from build123d import *

# Parameters (mm, degrees)
SKETCH1_W               = 20
SKETCH1_H               = 40
BOSS_EXTRUDE1_DEPTH     = 20
SKETCH2_W               = 13.1
SKETCH2_H               = 13.1
CUT_EXTRUDE1_DEPTH      = 49.989794856
SKETCH3_W               = 13.1
SKETCH3_H               = 13.1
CUT_EXTRUDE2_DEPTH      = 40.033447196
BOSS_EXTRUDE2_DEPTH     = 10
SKETCH5_W               = 20
SKETCH5_H               = 40
BOSS_EXTRUDE3_DEPTH     = 12
SKETCH6_W               = 13.1
SKETCH6_H               = 8
CUT_EXTRUDE3_DEPTH      = 13.1
SKETCH7_R               = 2
CUT_EXTRUDE4_DEPTH      = 55.990908339
CUT_EXTRUDE5_DEPTH      = 54.83216975
CUT_EXTRUDE5_DEPTH_BACK = 54.83216975
SKETCH8_R               = 2
CUT_EXTRUDE6_DEPTH      = 55.990908339


with BuildPart() as part:
    # Sketch1 → Boss-Extrude1 (new body)
    with BuildSketch(Plane(origin=(0, 0, 0), x_dir=(1, 0, 0), z_dir=(0, 1, 0))):
        with Locations((10, 20)):
            Rectangle(SKETCH1_W, SKETCH1_H)
    extrude(amount=BOSS_EXTRUDE1_DEPTH)

    # Sketch2 → Cut-Extrude1 (cut, through all)
    with BuildSketch(Plane(origin=(0, 20, 0), x_dir=(1, 0, 0), z_dir=(0, 1, 0))):
        with Locations((10, 6.55)):
            Rectangle(SKETCH2_W, SKETCH2_H)
    extrude(amount=-CUT_EXTRUDE1_DEPTH, mode=Mode.SUBTRACT)

    # Sketch3 → Cut-Extrude2 (cut, through all)
    with BuildSketch(Plane.XY.offset(-13.1)):
        with Locations((10, 13.45)):
            Rectangle(SKETCH3_W, SKETCH3_H)
    extrude(amount=-CUT_EXTRUDE2_DEPTH, mode=Mode.SUBTRACT)

    # Sketch4 → Boss-Extrude2 (add)
    with BuildSketch(Plane.XZ):
        Polygon((3.45, -13.1), (3.45, 0), (0, 0), (0, -40), (20, -40), (20, 0), (16.55, 0), (16.55, -13.1), align=None)
    extrude(amount=BOSS_EXTRUDE2_DEPTH)

    # Sketch5 → Boss-Extrude3 (add)
    with BuildSketch(Plane(origin=(0, 20, 0), x_dir=(1, 0, 0), z_dir=(0, 1, 0))):
        with Locations((10, 20)):
            Rectangle(SKETCH5_W, SKETCH5_H)
    extrude(amount=BOSS_EXTRUDE3_DEPTH)

    # Sketch6 → Cut-Extrude3 (cut)
    with BuildSketch(Plane.XY):
        with Locations((10, 24)):
            Rectangle(SKETCH6_W, SKETCH6_H)
    extrude(amount=-CUT_EXTRUDE3_DEPTH, mode=Mode.SUBTRACT)

    # Sketch7 → Cut-Extrude4 (cut, through all)
    with BuildSketch(Plane(origin=(20, 0, 0), x_dir=(0, 0, -1), z_dir=(1, 0, 0))):
        with Locations((6.55, -4)):
            Circle(SKETCH7_R)
        with Locations((6.55, 16)):
            Circle(SKETCH7_R)
        with Locations((6.55, 6)):
            Circle(SKETCH7_R)
    extrude(amount=-CUT_EXTRUDE4_DEPTH, mode=Mode.SUBTRACT)

    # Sketch8 → Cut-Extrude5 (cut, two sides: drawn at the far end of the back side and taken through both)
    with BuildSketch(Plane(origin=(3.45, 0, 0), x_dir=(0, 0, -1), z_dir=(1, 0, 0)).offset(-CUT_EXTRUDE5_DEPTH_BACK)):
        with Locations((34, 13.45)):
            Circle(SKETCH8_R)
        with Locations((26, 13.45)):
            Circle(SKETCH8_R)
        with Locations((18, 13.45)):
            Circle(SKETCH8_R)
    extrude(amount=CUT_EXTRUDE5_DEPTH + CUT_EXTRUDE5_DEPTH_BACK, mode=Mode.SUBTRACT)

    # Sketch9 → Cut-Extrude6 (cut, through all)
    with BuildSketch(Plane(origin=(20, 0, 0), x_dir=(0, 0, -1), z_dir=(1, 0, 0))):
        Polygon((18.1, -10), (40, -10), (40, 1.9), align=None)
    extrude(amount=-CUT_EXTRUDE6_DEPTH, mode=Mode.SUBTRACT)


solid = part.part
Verification items for the finished model (mm, model axes). A direction names the side the tool comes from. Give positions to 0.01 mm unless a question says otherwise; leave off trailing zeros. Loops run counter-clockwise (first coordinate to the right, second up) from the corner with the lowest first, then second, coordinate; pieces in that order, holes last. Notation, with made-up numbers: (-40, 82) - (-11, 82) arc R6 ccw to (-11, 86) - close; hole circle Ø1 at (81.5, 34). An arc over 180 degrees is marked (long way). Write item = value, one per line. Start each with the question number.
Q1. Tool access check on faces 4 (the face through (10, 6.9, -26)), 5 (the face through (3.45, 9, -16)), 6 (the face through (10, -1, -13.1)). Record the directions out of +Z, -Z, +X, -X, +Y, -Y that give a thin tool (end or side, any length) a straight path to the whole face; none if there is none.
Q2. Mould release check, pull along Z, two halves, no side actions. Record for faces 1 (the face through (8, -10, -15)), 2 (the face through (1.701, 14.051, -35.908)), 3 (the face through (10, 24, -13.1)): released by +Z, released by -Z, zero draft, split by the parting line, or undercut.
Q3. Thickness scan on line 1 (Y direction, x = 19.05, z = -6.55); line 2 (Z direction, x = 18.85, y = 13.45); line 3 (Y direction, x = 2.7, z = -18). Record the ranges inside material, lowest first.
Q4. Depth check by flat-ended pin: P1, Ø2.5, axis at x = 7, y = 22, coming from the +Z side. Enter the tip coordinate at first touch or a pass-through.
Q5. Cross-section at C-C, the plane z = -34. Enter the section's corners in (x, y), and give its area (3 significant figures).
Q6. Cross-section at A-A, the plane y = 13.45. State how many separate pieces and enclosed holes the cut face has, and give its area (3 significant figures).
Q7. Cross-section at B-B, the plane y = 6. Enter the section's corners in (x, z).
Answer key:
q1.face_4 = +Z, -Z
q1.face_5 = +Z
q1.face_6 = +Z, -Y
q2.face_1 = zero draft
q2.face_2 = undercut
q2.face_3 = released by +Z
q3.line_1 = -10 to -6, -2 to 4, 8 to 14, 18 to 32
q3.line_2 = -40 to -36, -32 to -28, -24 to -20, -16 to 0
q3.line_3 = -10 to 11.45, 15.45 to 32
q4.P1 = -13.1
q5.outline = (0, -1.36) - (20, -1.36) - (20, 11.45) - (16.55, 11.45) - (16.55, 6.9) - (3.45, 6.9) - (3.45, 11.45) - (0, 11.45) - close; (0, 15.45) - (3.45, 15.45) - (3.45, 20) - (16.55, 20) - (16.55, 15.45) - (20, 15.45) - (20, 32) - (0, 32) - close
q5.area = 468 mm^2
q6.separate_pieces = 8
q6.enclosed_holes = 0
q6.area = 193 mm^2
q7.outline = (0, -40) - (20, -40) - (20, -8.55) - (16.55, -8.55) - (16.55, -13.1) - (3.45, -13.1) - (3.45, -8.55) - (0, -8.55) - close; (0, -4.55) - (3.45, -4.55) - (3.45, 0) - (0, 0) - close; (16.55, -4.55) - (20, -4.55) - (20, 0) - (16.55, 0) - close
